from build123d import *

# Parameters (mm, degrees)
BOSS_EXTRUDE1_DEPTH      = 13.5
BOSS_EXTRUDE1_DEPTH_BACK = 13.5
BOSS_EXTRUDE2_START      = -30
BOSS_EXTRUDE2_DEPTH      = 10
FILLET3_R                = 2
BOSS_EXTRUDE3_DEPTH      = 38
FILLET4_R                = 5
FILLET5_R                = 5


with BuildPart() as part:
    # Sketch1 → Boss-Extrude1 (new, two sides: drawn at the far end of the back side and taken through both)
    with BuildSketch(Plane(origin=(0, 0, 0), x_dir=(1, 0, 0), z_dir=(0, 1, 0)).offset(-BOSS_EXTRUDE1_DEPTH_BACK)):
        with BuildLine():
            Line((0, 0), (46, 0))
            ThreePointArc((46, 0), (51.656854249, 2.343145751), (54, 8))
            Line((54, 8), (54, 68))
            Line((54, 68), (26, 68))
            Line((26, 68), (26, 35))
            ThreePointArc((26, 35), (24.535533906, 31.464466094), (21, 30))
            Line((21, 30), (0, 30))
            Line((0, 30), (0, 15))
            Line((0, 15), (0, 0))
        make_face()
    extrude(amount=BOSS_EXTRUDE1_DEPTH + BOSS_EXTRUDE1_DEPTH_BACK)

    # Sketch2 → Boss-Extrude2 (add)
    with BuildSketch(Plane.XY.offset(BOSS_EXTRUDE2_START)):
        with BuildLine():
            Line((0, -13.5), (-31.5, -13.5))
            ThreePointArc((-31.5, -13.5), (-44.299517979, 4.292125289), (-23.361165214, 10.770764519))
            ThreePointArc((-23.361165214, 10.770764519), (-21.936457993, 10.019374349), (-20.346781961, 9.759936564))
            Line((-20.346781961, 9.759936564), (0, 9.759936564))
            Line((0, 9.759936564), (0, -13.5))
        make_face()
    extrude(amount=BOSS_EXTRUDE2_DEPTH)

    # Fillet3
    fillet3_edges = [part.edges().sort_by_distance(p)[0] for p in [
        (0, 9.759936564, -25),
        (0, -1.870031718, -20),
    ]]
    fillet(fillet3_edges, radius=FILLET3_R)

    # Sketch4 → Boss-Extrude3 (add)
    with BuildSketch(Plane.ZY.offset(-26)):
        with BuildLine():
            ThreePointArc((-90, 15.5), (-105.482977781, -0.726222431), (-88.549150224, -15.431948514))
            Line((-88.549150224, -15.431948514), (-68, -13.5))
            Line((-68, -13.5), (-68, 13.5))
            Line((-68, 13.5), (-87.204918033, 15.245901639))
            Line((-87.204918033, 15.245901639), (-90, 15.5))
        make_face()
    extrude(amount=-BOSS_EXTRUDE3_DEPTH)

    # Fillet4
    fillet4_edges = [part.edges().sort_by_distance(p)[0] for p in [
        (54, 0, -68),
    ]]
    fillet(fillet4_edges, radius=FILLET4_R)

    # Fillet5
    fillet5_edges = [part.edges().sort_by_distance(p)[0] for p in [
        (64, 0, -68),
    ]]
    fillet(fillet5_edges, radius=FILLET5_R - 0.0001)  # a hair under: the kernel refuses the full size


solid = part.part
Verification items for the finished model (mm, model axes). A direction names the side the tool comes from. Round coordinates to 2 decimals unless told otherwise and drop trailing zeros. Loops run counter-clockwise (first coordinate to the right, second up) from the corner with the lowest first, then second, coordinate; pieces in that order, holes last. Notation, with made-up numbers: (-14, 21) - (27, 21) arc R25 ccw to (27, 40) - close; hole circle Ø11 at (1.25, 32.25). An arc over 180 degrees is marked (long way). Use a Markdown table: item, result. Add a question column.
1. Release check for a two-part mould opening along X. For faces 5 (the face through (-11, 9.76, -25)), 6 (the face through (-21.958, 10.027, -25.07)), 7 (the face through (64, 0, -89)), 8 (the face through (25, 0, -32)) record: released by +X, released by -X, zero draft, split by the parting line, or undercut.
2. Access from +Z, -Z, +X, -X, +Y, -Y to the whole of each face (thin tool, end or side, straight path). Record for faces 1 (the face through (54, 0, -35)), 2 (the face through (-23, 0, -20)), 3 (the face through (26, 0, -71)), 4 (the face through (24, -13.5, -27)).
3. Section check D-D, the plane x = -12. Record the boundary of the cut face in (y, z), plus the area to 3 significant figures.
4. Section check B-B, the plane x = 28. Record the boundary of the cut face in (y, z).
5. Thickness scan on probe 1 along Y at (x, z) = (34.5, -5.5); probe 2 along X at (y, z) = (2.5, -88); probe 3 along Z at (x, y) = (-30.5, -4). Record the ranges inside material, lowest first. Write a range as [from, to].
6. Section check C-C, the plane z = -36.5. Record the boundary of the cut face in (x, y), plus the area to 3 significant figures.
7. Gauge pin test, flat ends, axial feed: pin 1 (1.5 mm diameter, centred on y = 10, z = -31.5, fed in from -X); pin 2 (8 mm diameter, centred on x = -24.5, y = -3.5, fed in from -Z); pin 3 (1.5 mm diameter, centred on x = 20.5, z = -24.5, fed in from +Y). Record the tip position at first contact, or that the pin passes through.
Checks:
| question | item | result |
|---|---|---|
| 1 | face 5 | undercut |
| 1 | face 6 | undercut |
| 1 | face 7 | released by +X |
| 1 | face 8 | released by -X |
| 2 | face 1 | +Z, +X, +Y, -Y |
| 2 | face 2 | +Z, -X, +Y, -Y |
| 2 | face 3 | -Z, -X, +Y, -Y |
| 2 | face 4 | +Z, +X, -X, -Y |
| 3 | outline | (-13.5, -30) - (9.76, -30) - (9.76, -20) - (-13.5, -20) - close |
| 3 | area | 233 mm^2 |
| 4 | outline | (-15.43, -88.55) arc R15.5 ccw (long way) to (15.5, -90) - (13.5, -68) - (13.5, 0) - (-13.5, 0) - (-13.5, -68) - close |
| 5 | probe 1 | y = [-13.5, 13.5] |
| 5 | probe 2 | x = [26, 64] |
| 5 | probe 3 | z = [-30, -20] |
| 6 | outline | (26, -13.5) - (54, -13.5) - (54, 13.5) - (26, 13.5) - close |
| 6 | area | 756 mm^2 |
| 7 | pin 1 | stops at x = 23.63 |
| 7 | pin 2 | stops at z = -30 |
| 7 | pin 3 | stops at y = 13.5 |
